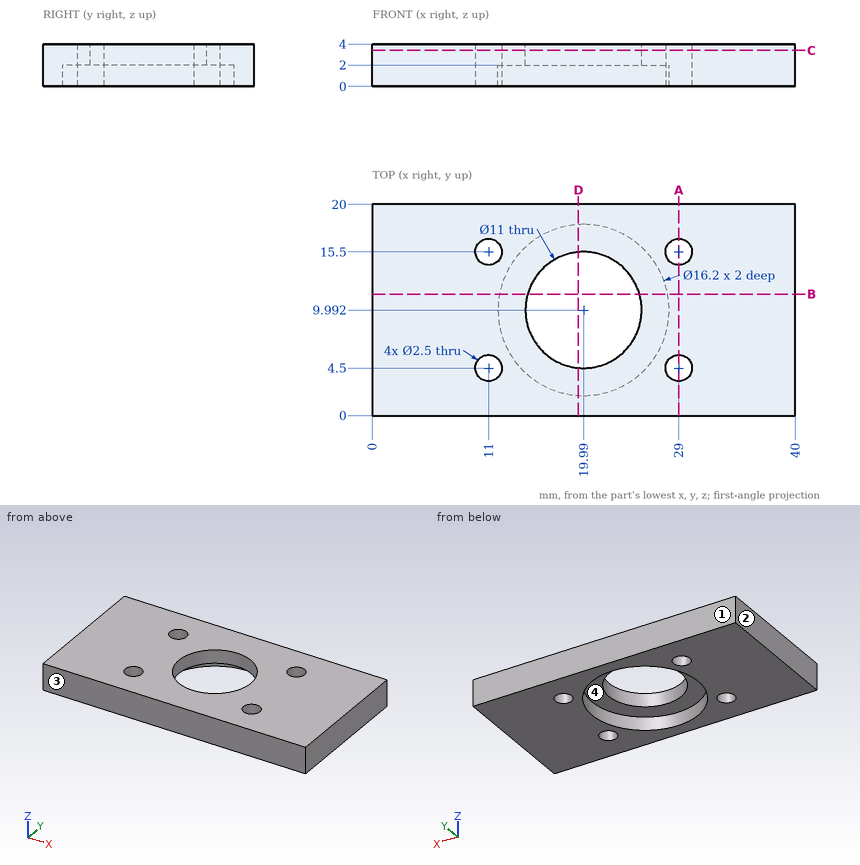
For this review, use the dimensioned drawing (mm, ordinates from the lowest corner) and the shaded views. Round coordinates to 2 decimals unless told otherwise and drop trailing zeros. Order: outer loops, then holes, each group sorted by start corner. A loop starts at its lowest first (then second) coordinate and runs counter-clockwise, first axis right, second up. Notation, with made-up numbers: (87.25, 24) -> (137.25, 24) arc R31 ccw to (137.25, 48) -> close; hole circle Ø2 at (1.5, 2.25). An arc over 180 degrees is marked (long way). Put each result on its own line as item: value.
Q1. Add section C-C on z = 3.4. Write out the cut boundary in (x, y), plus the area to 3 significant figures.
Check result:
outline: (0, 0) -> (40, 0) -> (40, 20) -> (0, 20) -> close; hole circle Ø2.5 at (11, 4.5); hole circle Ø2.5 at (11, 15.5); hole circle Ø11 at (19.99, 9.99); hole circle Ø2.5 at (29, 4.5); hole circle Ø2.5 at (29, 15.5)
area: 685 mm2
Q2. Add section D-D on x = 19.5. Write out the cut boundary in (y, z) (1 decimal).
Check result:
outline: (0, 0) -> (1.9, 0) -> (1.9, 2) -> (4.5, 2) -> (4.5, 4) -> (0, 4) -> close; (15.5, 2) -> (18.1, 2) -> (18.1, 0) -> (20, 0) -> (20, 4) -> (15.5, 4) -> close
Q3. For probe 1 along Y at (x, z) = (11, 1.2); probe 2 along X at (y, z) = (3.75, 0.85); probe 3 along Y at (x, z) = (25.5, 1.05) (1 decimal), list the stretches that pass through material, from the lowest coordinate up. Write a range as [from, to].
Check result:
probe 1: [0, 3.25], [5.75, 14.25], [16.75, 20]
probe 2: [0, 10], [12, 14.83], [25.15, 28], [30, 40]
probe 3: [0, 4.1], [15.9, 20]
Q4. Add section A-A on x = 29. Write out the cut boundary in (y, z).
Check result:
outline: (0, 0) -> (3.25, 0) -> (3.25, 4) -> (0, 4) -> close; (5.75, 0) -> (14.25, 0) -> (14.25, 4) -> (5.75, 4) -> close; (16.75, 0) -> (20, 0) -> (20, 4) -> (16.75, 4) -> close
Q5. Add section B-B on y = 11.5. Write out the cut boundary in (x, z), plus the area to 3 significant figures.
Check result:
outline: (0, 0) -> (12.03, 0) -> (12.03, 2) -> (14.7, 2) -> (14.7, 4) -> (0, 4) -> close; (25.28, 2) -> (27.95, 2) -> (27.95, 0) -> (40, 0) -> (40, 4) -> (25.28, 4) -> close
area: 107 mm2
Q6. Insertion check: pin 1 Ø2 at (x, y) = (11, 15.5) entering from -Z. The pin has a flat end and moves straight along its axis. Give the tip position at first contact, or say it passes through.
Check result:
pin 1: through
Q7. Mouldability with a two-part tool opening along Y and no side actions: class the marked faces 1, 2, 3 and 4 as pulls with the +Y half, pulls with the -Y half, needs draft (parallel to the pull), parting line crosses it, or undercut.
Check result:
face 1: pulls with the +Y half
face 2: needs draft
face 3: pulls with the -Y half
face 4: undercut
